```python
from build123d import *
from build123d.topology import SkipClean

# Parameters (mm, degrees)
SKETCH_1_R          = 1.65
SKETCH_1_R_2        = 5
SKETCH_1_R_3        = 4
EXTRUDE_1_DEPTH     = 3
CUT_EXTRUDE_1_DEPTH = 5
CUT_EXTRUDE_START   = -2
SKETCH_3_R          = 2.55
CUT_EXTRUDE_2_DEPTH = 1
SKETCH_4_R          = 20
EXTRUDE_2_DEPTH     = 3
SKETCH_5_R          = 11
SKETCH_5_R_2        = 1.65
SKETCH_5_R_3        = 2
CUT_EXTRUDE_3_DEPTH = 61.952850631
FILLET_1_R          = 3
SKETCH_8_R          = 7.5
EXTRUDE_4_DEPTH     = 0.25
SKETCH_9_R          = 7
SKETCH_9_R_2        = 5
CUT_EXTRUDE_4_DEPTH = 1
FILLET_2_R          = 1
SKETCH_11_R         = 7.5
CUT_EXTRUDE_6_DEPTH = 0.25


with BuildPart() as part:
    # 草图1 → 凸台-拉伸1 (new body)
    with BuildSketch(Plane.XY):
        with BuildLine():
            Line((1.82, -13.881195914), (50.975, -7.436354954))
            ThreePointArc((50.975, -7.436354954), (57.5, 0), (50.975, 7.436354954))
            Line((50.975, 7.436354954), (1.82, 13.881195914))
            ThreePointArc((1.82, 13.881195914), (-14, 0), (1.82, -13.881195914))
        make_face()
        with Locations((-9, 0)):
            Circle(SKETCH_1_R, mode=Mode.SUBTRACT)
        with Locations((4.5, 7.794228634)):
            Circle(SKETCH_1_R, mode=Mode.SUBTRACT)
        with Locations((4.5, -7.794228634)):
            Circle(SKETCH_1_R, mode=Mode.SUBTRACT)
        Circle(SKETCH_1_R_2, mode=Mode.SUBTRACT)
        with Locations((50, 0)):
            Circle(SKETCH_1_R_3, mode=Mode.SUBTRACT)
    extrude(amount=EXTRUDE_1_DEPTH)

    # 草图2 → 切除-拉伸1 (cut)
    with BuildSketch(Plane.XY.offset(3)):
        with BuildLine():
            Line((16.077054233, -5.960564335), (39.784103065, -2.852270991))
            ThreePointArc((39.784103065, -2.852270991), (40.77864829, -2.278773581), (41.076374055, -1.17))
            ThreePointArc((41.076374055, -1.17), (41, 0), (41.076374055, 1.17))
            ThreePointArc((41.076374055, 1.17), (40.77864829, 2.278773581), (39.784103065, 2.852270991))
            Line((39.784103065, 2.852270991), (16.077054233, 5.960564335))
            ThreePointArc((16.077054233, 5.960564335), (14.747754312, 5.454804266), (14.438231121, 4.066630313))
            ThreePointArc((14.438231121, 4.066630313), (15, 0), (14.438231121, -4.066630313))
            ThreePointArc((14.438231121, -4.066630313), (14.747754312, -5.454804266), (16.077054233, -5.960564335))
        make_face()
    extrude(amount=-CUT_EXTRUDE_1_DEPTH, mode=Mode.SUBTRACT)

    # 草图3 → 切除-拉伸2 (cut)
    with BuildSketch(Plane.XY.offset(3).offset(CUT_EXTRUDE_START)):
        with Locations((-9, 0)):
            Circle(SKETCH_3_R)
        with Locations((4.5, 7.794228634)):
            Circle(SKETCH_3_R)
        with Locations((4.5, -7.794228634)):
            Circle(SKETCH_3_R)
    extrude(amount=-CUT_EXTRUDE_2_DEPTH, mode=Mode.SUBTRACT)

    # 草图4 → 凸台-拉伸2 (add, through all)
    with BuildSketch(Plane.XY.offset(3)):
        Circle(SKETCH_4_R)
    extrude(amount=-EXTRUDE_2_DEPTH)

    # 草图5 → 切除-拉伸3 (cut, through all)
    with BuildSketch(Plane.XY.offset(3)):
        Circle(SKETCH_5_R)
        with Locations((-17.5, 0)):
            Circle(SKETCH_5_R_2)
        with Locations((8.75, 15.155444566)):
            Circle(SKETCH_5_R_2)
        with Locations((8.75, -15.155444566)):
            Circle(SKETCH_5_R_2)
        with Locations((-7.5, 12.990381057)):
            Circle(SKETCH_5_R_3)
        with Locations((15, 0)):
            Circle(SKETCH_5_R_3)
        with Locations((-7.5, -12.990381057)):
            Circle(SKETCH_5_R_3)
    extrude(amount=-CUT_EXTRUDE_3_DEPTH, mode=Mode.SUBTRACT)

    # 圆角1
    fillet_1_edges = [part.edges().sort_by_distance(p)[0] for p in [
        (15.981652446, -12.024424522, 1.5),
        (19.214751718, -5.549172589, 1.5),
        (15.981652446, 12.024424522, 1.5),
        (19.214751718, 5.549172589, 1.5),
    ]]
    fillet(fillet_1_edges, radius=FILLET_1_R)

    # 草图8 → 凸台-拉伸4 (add)
    with SkipClean():  # the faces are left unmerged after this step: merging them gives an invalid solid
        with BuildSketch(Plane(origin=(0, 0, 3), x_dir=(-1, 0, 0), z_dir=(0, 0, -1))):
            with Locations((-50, 0)):
                Circle(SKETCH_8_R)
        extrude(amount=-EXTRUDE_4_DEPTH)

    # 草图9 → 切除-拉伸4 (cut)
    with SkipClean():  # the faces are left unmerged after this step: merging them gives an invalid solid
        with BuildSketch(Plane.XY.offset(3.25)):
            with Locations((50, 0)):
                Circle(SKETCH_9_R)
            with Locations((50, 0)):
                Circle(SKETCH_9_R_2, mode=Mode.SUBTRACT)
        extrude(amount=-CUT_EXTRUDE_4_DEPTH, mode=Mode.SUBTRACT)

    # 圆角2
    fillet_2_edges = [part.edges().sort_by_distance(p)[0] for p in [
        (43, 0, 2.25),
        (45, 0, 2.25),
    ]]
    fillet(fillet_2_edges, radius=FILLET_2_R - 0.0001)  # a hair under: the kernel refuses the full size

    # 草图11 → 切除-拉伸6 (cut)
    with BuildSketch(Plane(origin=(0, 0, 3), x_dir=(-1, 0, 0), z_dir=(0, 0, -1))):
        with Locations((-50, 0)):
            Circle(SKETCH_11_R)
    extrude(amount=-CUT_EXTRUDE_6_DEPTH, mode=Mode.SUBTRACT)


solid = part.part
```
Part model, mm, in its own coordinate system. A direction names the side the tool comes from. Coordinates: 2 decimals unless noted, no trailing zeros. Write each loop counter-clockwise with the first axis right and the second up, starting at its lowest first coordinate (ties: lowest second). Pieces come first, ordered by that corner, then holes.
Item 1: Slice it at B-B (y = 0). Count the separate pieces of the cut face and the enclosed holes in it, and give its area (3 significant figures).
Item 2: Probe line 1 (Y direction, x = -7.5, z = 2.2); line 2 (Y direction, x = 8.75, z = 1.8); line 3 (Y direction, x = -0.5, z = 2.6). List the from-to ranges inside material, lowest first.
Item 3: Pin check, flat tips, straight feed: pin 1 (3 mm diameter, centred on x = 15, y = 0, fed in from -Z); pin 2 (1 mm diameter, centred on x = 27, z = 0.5, fed in from -Y). Stop position of each tip, or through.
Item 4: Slice it at D-D (x = 8.75). Write the cut outline in (y, z).
Item 5: Slice it at A-A (x = 0). Write the cut outline in (y, z).
Item 6: Mould opens along Y. For faces 1 (the face through (33.841, -9.683, 1.479)), 2 (the face through (11, 5, 3)), 3 (the face through (-9.087, -14.207, 1.521)) say: released by +Y, released by -Y, zero draft, split by the parting line, or undercut.
Item 7: Which spindle directions (+Z, -Z, +X, -X, +Y, -Y) get a long thin tool onto all of the face, cutting with end or side? Do faces 4 (the face through (34.31, 9.62, 1.48)), 5 (the face through (31.426, -3.948, 1.521)). Say none if no direction does.
Results found:
1. separate pieces: 6
1. enclosed holes: 0
1. area: 55.4 mm2
2. line 1: y = -18.54 to -14.99, -10.99 to -8.05, 8.05 to 10.99, 14.99 to 18.54
2. line 2: y = -17.98 to -16.81, -13.51 to -6.67, 6.67 to 13.51, 16.81 to 17.98
2. line 3: y = -19.99 to -10.99, 10.99 to 19.99
3. pin 1: passes through
3. pin 2: stops at y = -10.65
4. outline: (-17.98, 0) - (-16.81, 0) - (-16.81, 3) - (-17.98, 3) - close; (-13.51, 0) - (-6.67, 0) - (-6.67, 3) - (-13.51, 3) - close; (6.67, 0) - (13.51, 0) - (13.51, 3) - (6.67, 3) - close; (16.81, 0) - (17.98, 0) - (17.98, 3) - (16.81, 3) - close
5. outline: (-20, 0) - (-11, 0) - (-11, 3) - (-20, 3) - close; (11, 0) - (20, 0) - (20, 3) - (11, 3) - close
6. face 1: released by -Y
6. face 2: zero draft
6. face 3: undercut
7. face 4: +Z, -Z, +X, +Y
7. face 5: +Z, -Z
